Here's how the part is built. I have some questions about the finished solid (model axes, mm). A direction names the side the tool comes from. Give positions to 0.01 mm unless a question says otherwise; leave off trailing zeros. Loops run counter-clockwise (first coordinate to the right, second up) from the corner with the lowest first, then second, coordinate; pieces in that order, holes last. Notation, with made-up numbers: M 0.5,23.25 L 42.5,23.25 A10 ccw 42.5,29.25 Z; hole C 15.5,-7.75 d9. An arc over 180 degrees is marked long. Write item = value, one per line. Start each with the question number.
Autodesk Inventor part; units mm, degrees
ref_plane "YZ Plane" through (0, 0, 0) normal (1, 0, 0) x (0, 1, 0)
ref_plane "XZ Plane" through (0, 0, 0) normal (0, 1, 0) x (-1, 0, 0)
ref_plane "XY Plane" through (0, 0, 0) normal (0, 0, 1) x (1, 0, 0)
sketch "Sketch1" plane through (0, 0, 0) normal (0, 0, 1) x (1, 0, 0)
  line L0 (0, 0) -> (20, 0)
  line L1 (20, 0) -> (20, 1)
  line L2 (20, 1) -> (1, 20)
  line L3 (1, 20) -> (0, 20)
  line L4 (0, 20) -> (0, 0)
  dimension "d0" = 135
  dimension "d1" = 20
  dimension "d2" = 20
  dimension "d3" = 1
extrude "Extrusion1" add sketch "Sketch1" along normal mid plane 20
sketch "Sketch2" plane through (0, 0, 10) normal (0, -1, 0) x (1, 0, 0)
  circle A0 centre (10, -10) radius 2.5
  point P0 (0, -10)
  dimension "d6" = 5
extrude "Extrusion2" cut sketch "Sketch2" against normal blind 3.5
sketch "Sketch3" plane through (10, 3.5, 0) normal (0, -1, 0) x (1, 0, 0)
  circle A0 centre (0, 0) radius 2.5
  circle A1 centre (0, 0) radius 5.5
  point P0 (-10, 0)
  dimension "d9" = 11
extrude "Extrusion3" cut sketch "Sketch3" against normal up to next contours A0 | A1
sketch "Sketch4" plane through (0, 0, 10) normal (-1, 0, 0) x (0, 0, 1)
  circle A0 centre (-10, 10) radius 2.5
  point P0 (-10, 0)
  dimension "d12" = 5
extrude "Extrusion4" cut sketch "Sketch4" against normal blind 3.5
sketch "Sketch5" plane through (3.5, 10, 0) normal (-1, 0, 0) x (0, 0, 1)
  circle A0 centre (0, 0) radius 2.5
  circle A1 centre (0, 0) radius 5.5
  point P0 (0, -10)
  dimension "d15" = 11
extrude "Extrusion5" cut sketch "Sketch5" against normal up to next contours A0 | A1
properties part number "Black Angle Corner Connector"
Q1. Will these pins go through, and if not, where does the flat tip stop? pin 1 (3 mm diameter, centred on x = 9, z = 2.5, fed in from +Y); pin 2 (5 mm diameter, centred on y = 5, z = 4.5, fed in from +X); pin 3 (10 mm diameter, centred on y = 9, z = 0, fed in from +X); pin 4 (4 mm diameter, centred on x = 10, z = 0, fed in from -Y).
Q2. If I drill on line 1 along Z through (x, y) = (7.5, 10); line 2 along X through (y, z) = (11.5, 4), over which ranges is the centre line in solid material (lowest first)?
Q3. If we section it at C-C, the plane z = 7.25: List the corners of the cut face in (x, y) for me.
Q4. If we section it at D-D, the plane y = 13: List the corners of the cut face in (x, z) for me, then the cut area to 3 significant figures.
Q5. If we section it at B-B, the plane y = 11: List the corners of the cut face in (x, z) for me.
Q6. We'd pull the mould along X, two halves only. Please class faces 4 (the cylindrical face through (1.73, 7.56, -0.54)), 5 (the cylindrical face through (5.26, 13.72, -4.05)), 6 (the cylindrical face through (12.82, 7.1, 4.72)), 7 (the flat face through (0, 12, 2)): pulls with the +X half, pulls with the -X half, needs draft (parallel to the pull), parting line crosses it, or undercut.
Q7. On a 3-axis mill with a long thin cutter (end or side, diameter ignored), from which of +Z, -Z, +X, -X, +Y, -Y can I reach the whole of each face in a straight line? I mean faces 1 (the cylindrical face through (7.5, 1.7, 0.1)), 2 (the flat face through (3.5, 13, 0)), 3 (the flat face through (10, 3.5, 3)). Say none if no direction works.
Q8. If we section it at A-A, the plane z = 0: List the corners of the cut face in (x, y) for me.
Resolved:
q1.pin_1 = 3.5
q1.pin_2 = 18.5
q1.pin_3 = 17
q1.pin_4 = through
q2.line_1 = -10 to -5.5, 5.5 to 10
q2.line_2 = 0 to 3.5
q3.outline = M 0,0 L 20,0 L 20,1 L 1,20 L 0,20 Z
q4.outline = M 0,-10 L 8,-10 L 8,-5.12 A5.5 cw 7,-4.61 L 3.5,-4.61 L 3.5,4.61 L 7,4.61 A5.5 cw 8,5.12 L 8,10 L 0,10 Z
q4.area = 118 mm²
q5.outline = M 0,-10 L 10,-10 L 10,-5.5 A5.5 cw 9,-5.41 L 3.5,-5.41 L 3.5,-2.29 L 0,-2.29 Z; M 0,2.29 L 3.5,2.29 L 3.5,5.41 L 9,5.41 A5.5 cw 10,5.5 L 10,10 L 0,10 Z
q6.face_4 = needs draft
q6.face_5 = undercut
q6.face_6 = undercut
q6.face_7 = pulls with the -X half
q7.face_1 = +Y, -Y
q7.face_2 = none
q7.face_3 = +Y
q8.outline = M 0,0 L 7.5,0 L 7.5,3.5 L 4.5,3.5 L 4.5,4.5 L 3.5,4.5 L 3.5,7.5 L 0,7.5 Z; M 0,12.5 L 3.5,12.5 L 3.5,15.5 L 4.5,15.5 L 4.5,16.5 L 1,20 L 0,20 Z; M 12.5,0 L 20,0 L 20,1 L 15.5,5.5 L 15.5,3.5 L 12.5,3.5 Z
